from build123d import *

# Parameters (mm, degrees)
SKETCH_1_W          = 24.72
SKETCH_1_H          = 49.22
EXTRUDE_1_DEPTH     = 36
SKETCH_3_W          = 24.72
SKETCH_3_H          = 32
CUT_EXTRUDE_1_DEPTH = 46.22
SKETCH_4_R          = 1
SKETCH_4_R_2        = 10
SKETCH_4_W          = 20.72
SKETCH_4_H          = 20.22
CUT_EXTRUDE_2_DEPTH = 2
SKETCH_6_R          = 1
CUT_EXTRUDE_3_DEPTH = 6
SKETCH_7_R          = 9.5
EXTRUDE_2_DEPTH     = 5
SKETCH_8_R          = 1.5
CUT_EXTRUDE_4_DEPTH = 8
FILLET_5_R          = 1
FILLET_6_R          = 1
FILLET_7_R          = 1
FILLET_8_R          = 1
FILLET_9_R          = 1
FILLET_10_R         = 1
SKETCH_9_R          = 3
CUT_EXTRUDE_5_DEPTH = 10
SKETCH_10_R         = 3
CUT_EXTRUDE_6_DEPTH = 2


with BuildPart() as part:
    # 草图1 → 凸台-拉伸1 (new body)
    with BuildSketch(Plane.XY):
        with Locations((12.36, 24.61)):
            Rectangle(SKETCH_1_W, SKETCH_1_H)
    extrude(amount=EXTRUDE_1_DEPTH)

    # 草图3 → 切除-拉伸1 (cut)
    with BuildSketch(Plane.XZ):
        with Locations((12.36, 18)):
            Rectangle(SKETCH_3_W, SKETCH_3_H)
    extrude(amount=-CUT_EXTRUDE_1_DEPTH, mode=Mode.SUBTRACT)

    # 草图4 → 切除-拉伸2 (cut)
    with BuildSketch(Plane.XY.offset(2)):
        with Locations((2, 2.36)):
            Circle(SKETCH_4_R)
        with Locations((22.72, 2.36)):
            Circle(SKETCH_4_R)
        with Locations((22.72, 26.81)):
            Circle(SKETCH_4_R)
        with Locations((2, 26.81)):
            Circle(SKETCH_4_R)
        with Locations((12.36, 36.11)):
            Circle(SKETCH_4_R_2)
        with Locations((12.36, 14.11)):
            Rectangle(SKETCH_4_W, SKETCH_4_H)
    extrude(amount=-CUT_EXTRUDE_2_DEPTH, mode=Mode.SUBTRACT)

    # 草图6 → 切除-拉伸3 (cut)
    with BuildSketch(Plane.XY.offset(36)):
        with BuildLine():
            Line((5.4, 27.996527822), (5.4, 28))
            Line((5.4, 28), (19.4, 28))
            Line((19.4, 28), (19.4, 27.940836898))
            ThreePointArc((19.4, 27.940836898), (21.640245754, 31.218722824), (22.428407613, 35.11))
            ThreePointArc((22.428407613, 35.11), (8.573804918, 44.337244337), (5.4, 27.996527822))
        make_face()
        with BuildLine():
            Line((19.4, 28), (5.4, 28))
            Line((5.4, 28), (5.4, 27.996527822))
            ThreePointArc((5.4, 27.996527822), (12.388628696, 25.110079118), (19.4, 27.940836898))
            Line((19.4, 27.940836898), (19.4, 28))
        make_face()
        with BuildLine():
            ThreePointArc((19.4, 27.940836898), (12.388628696, 25.110079118), (5.4, 27.996527822))
            Line((5.4, 27.996527822), (5.4, 0))
            Line((5.4, 0), (19.4, 0))
            Line((19.4, 0), (19.4, 27.940836898))
        make_face()
        with Locations((2, 26.81)):
            Circle(SKETCH_6_R)
        with Locations((22.72, 6.11)):
            Circle(SKETCH_6_R)
        with Locations((2, 6.11)):
            Circle(SKETCH_6_R)
        with Locations((22.72, 26.81)):
            Circle(SKETCH_6_R)
    extrude(amount=-CUT_EXTRUDE_3_DEPTH, mode=Mode.SUBTRACT)

    # 草图7 → 凸台-拉伸2 (add)
    with BuildSketch(Plane(origin=(0, 49.22, 0), x_dir=(1, 0, 0), z_dir=(0, 1, 0))):
        with Locations(Location((12.36, -20, 0), (0, 0, 270))):
            Circle(SKETCH_7_R)
    extrude(amount=EXTRUDE_2_DEPTH)

    # 草图8 → 切除-拉伸4 (cut)
    with BuildSketch(Plane(origin=(0, 54.22, 0), x_dir=(1, 0, 0), z_dir=(0, 1, 0))):
        with Locations(Location((12.36, -13, 0), (0, 0, 270))):
            Circle(SKETCH_8_R)
        with Locations(Location((12.36, -27, 0), (0, 0, 270))):
            Circle(SKETCH_8_R)
        with Locations(Location((19.36, -20, 0), (0, 0, 270))):
            Circle(SKETCH_8_R)
        with Locations(Location((5.36, -20, 0), (0, 0, 270))):
            Circle(SKETCH_8_R)
    extrude(amount=-CUT_EXTRUDE_4_DEPTH, mode=Mode.SUBTRACT)

    # 圆角5
    fillet_5_edges = [part.edges().sort_by_distance(p)[0] for p in [
        (0, 24.61, 36),
    ]]
    fillet(fillet_5_edges, radius=FILLET_5_R - 0.0001)  # a hair under: the kernel refuses the full size

    # 圆角6
    fillet_6_edges = [part.edges().sort_by_distance(p)[0] for p in [
        (24.72, 24.61, 36),
    ]]
    fillet(fillet_6_edges, radius=FILLET_6_R - 0.0001)  # a hair under: the kernel refuses the full size

    # 圆角7
    fillet_7_edges = [part.edges().sort_by_distance(p)[0] for p in [
        (0, 24.61, 0),
    ]]
    fillet(fillet_7_edges, radius=FILLET_7_R - 0.0001)  # a hair under: the kernel refuses the full size

    # 圆角8
    fillet_8_edges = [part.edges().sort_by_distance(p)[0] for p in [
        (24.72, 24.61, 0),
    ]]
    fillet(fillet_8_edges, radius=FILLET_8_R - 0.0001)  # a hair under: the kernel refuses the full size

    # 圆角9
    fillet_9_edges = [part.edges().sort_by_distance(p)[0] for p in [
        (19.4, 13.970418449, 34),
    ]]
    fillet(fillet_9_edges, radius=FILLET_9_R)

    # 圆角10
    fillet_10_edges = [part.edges().sort_by_distance(p)[0] for p in [
        (5.4, 13.998263911, 34),
    ]]
    fillet(fillet_10_edges, radius=FILLET_10_R)

    # 草图9 → 切除-拉伸5 (cut)
    with BuildSketch(Plane(origin=(0, 54.22, 0), x_dir=(1, 0, 0), z_dir=(0, 1, 0))):
        with Locations(Location((12.36, -20, 0), (0, 0, 270))):
            Circle(SKETCH_9_R)
    extrude(amount=-CUT_EXTRUDE_5_DEPTH, mode=Mode.SUBTRACT)

    # 草图10 → 切除-拉伸6 (cut)
    with BuildSketch(Plane.XZ.offset(-46.22)):
        with Locations(Location((12.36, 27, 0), (0, 0, 270))):
            Circle(SKETCH_10_R)
        with Locations(Location((5.36, 20, 0), (0, 0, 270))):
            Circle(SKETCH_10_R)
        with Locations(Location((12.36, 13, 0), (0, 0, 270))):
            Circle(SKETCH_10_R)
        with Locations(Location((19.36, 20, 0), (0, 0, 270))):
            Circle(SKETCH_10_R)
    extrude(amount=-CUT_EXTRUDE_6_DEPTH, mode=Mode.SUBTRACT)


solid = part.part
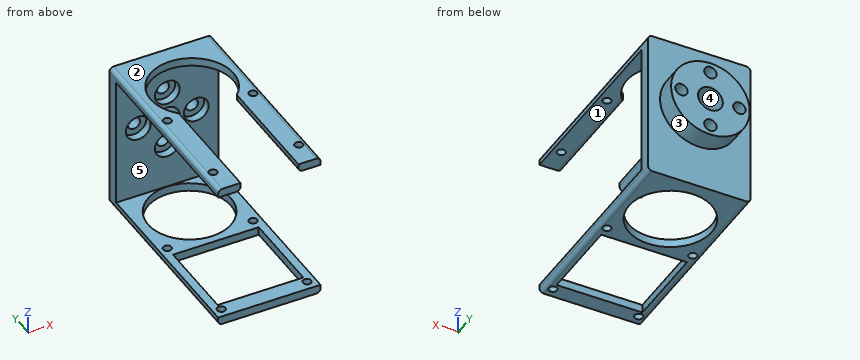
Build history of the part. All positions in model axes, mm. Face numbers are marked on the shaded views. A direction names the side the tool comes from. Round coordinates to 2 decimals unless told otherwise and drop trailing zeros. Write each loop counter-clockwise with the first axis right and the second up, starting at its lowest first coordinate (ties: lowest second). Pieces come first, ordered by that corner, then holes. Notation, with made-up numbers: (70.5, 62.5) -> (121.5, 62.5) arc R17 cw to (121.5, 76.5) -> close; hole circle Ø10 at (-33.5, 6). An arc over 180 degrees is marked (long way). Write item = value, one per line.
(1) Flat gauge pins, fed straight in: pin 1 (2.5 mm diameter, centred on x = 22.72, y = 26.81, fed in from -Z); pin 2 (1.6 mm diameter, centred on x = 22.72, y = 26.81, fed in from -Z); pin 3 (4 mm diameter, centred on x = 14, z = 32, fed in from +Y); pin 4 (3.5 mm diameter, centred on x = 12.36, z = 27, fed in from -Y). Where does each tip first touch, or does it go through?
Answer:
pin_1 = 0
pin_2 = through
pin_3 = 49.22
pin_4 = 48.22
(2) Band-saw the part on A-A (y = 6.11). State how many separate pieces and enclosed holes the cut face has, then the cut area to 3 significant figures.
Answer:
separate_pieces = 6
enclosed_holes = 0
area = 20.2 mm2
(3) Band-saw the part on D-D (z = 27.5). Give the cut face in (x, y).
Answer:
outline = (0, 46.22) -> (9.4, 46.22) -> (9.4, 48.22) -> (10.95, 48.22) -> (10.95, 54.22) -> (6.53, 54.22) -> (6.53, 49.22) -> (0, 49.22) -> close; (13.77, 48.22) -> (15.32, 48.22) -> (15.32, 46.22) -> (24.72, 46.22) -> (24.72, 49.22) -> (18.19, 49.22) -> (18.19, 54.22) -> (13.77, 54.22) -> close
(4) Two-plate mould, pull along X, no slides. Class the marked faces 3, 4 and 5: pulls with the +X half, pulls with the -X half, needs draft (parallel to the pull), parting line crosses it, or undercut.
Answer:
face_3 = parting line crosses it
face_4 = undercut
face_5 = needs draft
(5) Tool access for the marked faces 1 and 2: list every direction of +Z, -Z, +X, -X, +Y, -Y with a clear straight run to the whole face (end or side of a thin tool).
Answer:
face_1 = +X, -X, -Y
face_2 = +Z, +X, -X, +Y, -Y
(6) Band-saw the part on C-C (y = 20). Give the cut face in (x, z).
Answer:
outline = (0, 1) arc R1 ccw to (1, 0) -> (2, 0) -> (2, 2) -> (0, 2) -> close; (0, 34) -> (4.4, 34) arc R1 ccw to (5.4, 35) -> (5.4, 36) -> (1, 36) arc R1 ccw to (0, 35) -> close; (19.4, 35) arc R1 ccw to (20.4, 34) -> (24.72, 34) -> (24.72, 35) arc R1 ccw to (23.72, 36) -> (19.4, 36) -> close; (22.72, 0) -> (23.72, 0) arc R1 ccw to (24.72, 1) -> (24.72, 2) -> (22.72, 2) -> close
(7) Band-saw the part on B-B (z = 20). Give the cut face in (x, y).
Answer:
outline = (0, 46.22) -> (2.36, 46.22) -> (2.36, 48.22) -> (3.86, 48.22) -> (3.86, 54.22) -> (2.86, 54.22) -> (2.86, 49.22) -> (0, 49.22) -> close; (6.86, 48.22) -> (8.36, 48.22) -> (8.36, 46.22) -> (9.36, 46.22) -> (9.36, 54.22) -> (6.86, 54.22) -> close; (15.36, 46.22) -> (16.36, 46.22) -> (16.36, 48.22) -> (17.86, 48.22) -> (17.86, 54.22) -> (15.36, 54.22) -> close; (20.86, 48.22) -> (22.36, 48.22) -> (22.36, 46.22) -> (24.72, 46.22) -> (24.72, 49.22) -> (21.86, 49.22) -> (21.86, 54.22) -> (20.86, 54.22) -> close
(8) Probe L1, parallel to X at y = 47.15, z = 20; L2, parallel to X at y = 49.5, z = 20; L3, parallel to Z at x = 3.25, y = 2.5. List the from-to ranges inside material, lowest first.
Answer:
L1 = 0 to 2.36, 8.36 to 9.36, 15.36 to 16.36, 22.36 to 24.72
L2 = 2.86 to 3.86, 6.86 to 9.36, 15.36 to 17.86, 20.86 to 21.86
L3 = 0 to 2, 34 to 36
